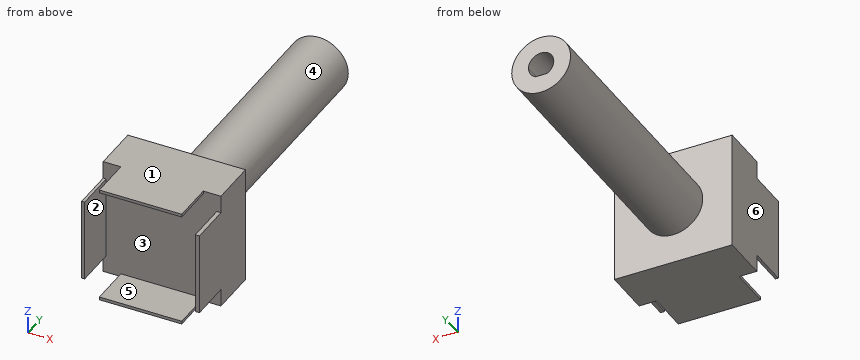
```python
from build123d import *

# Parameters (mm, degrees)
SKETCH_1_W          = 20
SKETCH_1_H          = 20
SKETCH_1_W_2        = 18.8
SKETCH_1_H_2        = 19
EXTRUDE_1_DEPTH     = 7
SKETCH_3_W          = 20
SKETCH_3_H          = 20
EXTRUDE_2_DEPTH     = 8
SKETCH_4_R          = 5
EXTRUDE_3_DEPTH     = 43
CUT_EXTRUDE_1_DEPTH = 18
SKETCH_6_W          = 3
SKETCH_6_H          = 3
CUT_EXTRUDE_2_DEPTH = 10


with BuildPart() as part:
    # 草圖1 → 填料-伸長1 (new body)
    with BuildSketch(Plane(origin=(0, 0, 0), x_dir=(1, 0, 0), z_dir=(0, 1, 0))):
        with Locations((10, 10)):
            Rectangle(SKETCH_1_W, SKETCH_1_H)
        with Locations((9.9, 10)):
            Rectangle(SKETCH_1_W_2, SKETCH_1_H_2, mode=Mode.SUBTRACT)
    extrude(amount=EXTRUDE_1_DEPTH)

    # 草圖3 → 填料-伸長2 (add)
    with BuildSketch(Plane(origin=(0, 7, 0), x_dir=(1, 0, 0), z_dir=(0, 1, 0))):
        with Locations((10, 10)):
            Rectangle(SKETCH_3_W, SKETCH_3_H)
    extrude(amount=EXTRUDE_2_DEPTH)

    # 草圖4 → 填料-伸長3 (add)
    with BuildSketch(Plane(origin=(0, 15, 0), x_dir=(1, 0, 0), z_dir=(0, 1, 0))):
        with Locations((10, 10)):
            Circle(SKETCH_4_R)
    extrude(amount=EXTRUDE_3_DEPTH)

    # 草圖5 → 除料-伸長1 (cut)
    with BuildSketch(Plane(origin=(0, 58, 0), x_dir=(1, 0, 0), z_dir=(0, 1, 0))):
        with BuildLine():
            Line((10, 11.9), (8.99376941, 11.9))
            ThreePointArc((8.99376941, 11.9), (8.891148289, 8.158004375), (12.15, 10))
            ThreePointArc((12.15, 10), (11.841995625, 11.108851711), (11.00623059, 11.9))
            Line((11.00623059, 11.9), (10, 11.9))
        make_face()
    extrude(amount=-CUT_EXTRUDE_1_DEPTH, mode=Mode.SUBTRACT)

    # 草圖6 → 除料-伸長2 (cut)
    with BuildSketch(Plane(origin=(0, 7, 0), x_dir=(1, 0, 0), z_dir=(0, 1, 0))):
        with Locations((1.5, 18.5)):
            Rectangle(SKETCH_6_W, SKETCH_6_H)
        with Locations((18.5, 18.5)):
            Rectangle(SKETCH_6_W, SKETCH_6_H)
        with Locations((18.5, 1.5)):
            Rectangle(SKETCH_6_W, SKETCH_6_H)
        with Locations((1.5, 1.5)):
            Rectangle(SKETCH_6_W, SKETCH_6_H)
    extrude(amount=-CUT_EXTRUDE_2_DEPTH, mode=Mode.SUBTRACT)


solid = part.part
```
The model under review builds one solid part; all positions refer to its coordinate system, in mm. Face numbers are marked on the shaded views. A direction names the side the tool comes from. Round coordinates to 2 decimals unless told otherwise and drop trailing zeros. Loops run counter-clockwise (first coordinate to the right, second up) from the corner with the lowest first, then second, coordinate; pieces in that order, holes last. Notation, with made-up numbers: (12.25, 3) - (32.25, 3) arc R28 cw to (32.25, 24) - close; hole circle Ø5 at (56.5, 1.25). An arc over 180 degrees is marked (long way). Use a Markdown table: item, result. Add a question column.
Q1. Add section B-B (y = 51). State the section outline as (x, z) points.
Q2. The part is to be moulded in two halves that separate along Z. For the marked faces 1, 2 and 3, say which applies: pulls with the +Z half, pulls with the -Z half, needs draft (parallel to the pull), parting line crosses it, or undercut.
Q3. Add section A-A (x = 10). State the section outline as (y, z) points, plus the area to 3 significant figures.
Q4. Machinability: for the marked faces 4, 5 and 6, which of the approach directions +Z, -Z, +X, -X, +Y, -Y give a long, thin tool a straight path to every point of the face, cutting with its end or side? Answer none if there is none.
Q5. For probe 1 along Z at (x, y) = (10, 54.5); probe 2 along Y at (x, z) = (18.5, -1.5); probe 3 along X at (y, z) = (46.5, -10), list the stretches that pass through material, from the lowest coordinate up.
Q6. Add section C-C (z = -8.5). State the section outline as (x, y) points.
Q7. Insertion check: pin 1 Ø5 at (x, z) = (10, -10) entering from -Y; pin 2 Ø0.6 at (y, z) = (2.5, -0.5) entering from -X; pin 3 Ø6 at (y, z) = (28.5, -11) entering from +X. Each pin has a flat end and moves straight along its axis. Give the tip position at first contact, or say it passes through.
Q8. Add section D-D (x = 15.75). State the section outline as (y, z) points.
Worked answers:
| question | item | result |
|---|---|---|
| 1 | outline | circle Ø10 at (10, -10); hole (8.99, -11.9) - (11.01, -11.9) arc R2.15 ccw (long way) to start |
| 2 | face 1 | pulls with the +Z half |
| 2 | face 2 | needs draft |
| 2 | face 3 | undercut |
| 3 | outline | (0, -20) - (15, -20) - (15, -15) - (58, -15) - (58, -11.9) - (40, -11.9) - (40, -7.85) - (58, -7.85) - (58, -5) - (15, -5) - (15, 0) - (0, 0) - (0, -0.5) - (7, -0.5) - (7, -19.5) - (0, -19.5) - close |
| 3 | area | 524 mm² |
| 4 | face 4 | +Y |
| 4 | face 5 | +X, -X, -Y |
| 4 | face 6 | +Z, -Z, -X, +Y, -Y |
| 5 | probe 1 | -15 to -11.9, -7.85 to -5 |
| 5 | probe 2 | 7 to 15 |
| 5 | probe 3 | 5 to 7.85, 12.15 to 15 |
| 6 | outline | (0, 0) - (0.5, 0) - (0.5, 7) - (19.3, 7) - (19.3, 0) - (20, 0) - (20, 15) - (14.77, 15) - (14.77, 58) - (11.54, 58) - (11.54, 40) - (8.46, 40) - (8.46, 58) - (5.23, 58) - (5.23, 15) - (0, 15) - close |
| 7 | pin 1 | y = 7 |
| 7 | pin 2 | x = 3 |
| 7 | pin 3 | x = 15 |
| 8 | outline | (0, -20) - (15, -20) - (15, 0) - (0, 0) - (0, -0.5) - (7, -0.5) - (7, -19.5) - (0, -19.5) - close |
